For this review, use the dimensioned drawing (mm, ordinates from the lowest corner) and the shaded views. A direction names the side the tool comes from. Round coordinates to 2 decimals unless told otherwise and drop trailing zeros. Write each loop counter-clockwise with the first axis right and the second up, starting at its lowest first coordinate (ties: lowest second). Pieces come first, ordered by that corner, then holes. Notation, with made-up numbers: M 78.25,33.5 L 129.25,33.5 A11 cw 129.25,54.5 Z; hole C 25.5,14 d6. An arc over 180 degrees is marked long. Use CSV: the item, a comma, the result in double quotes.
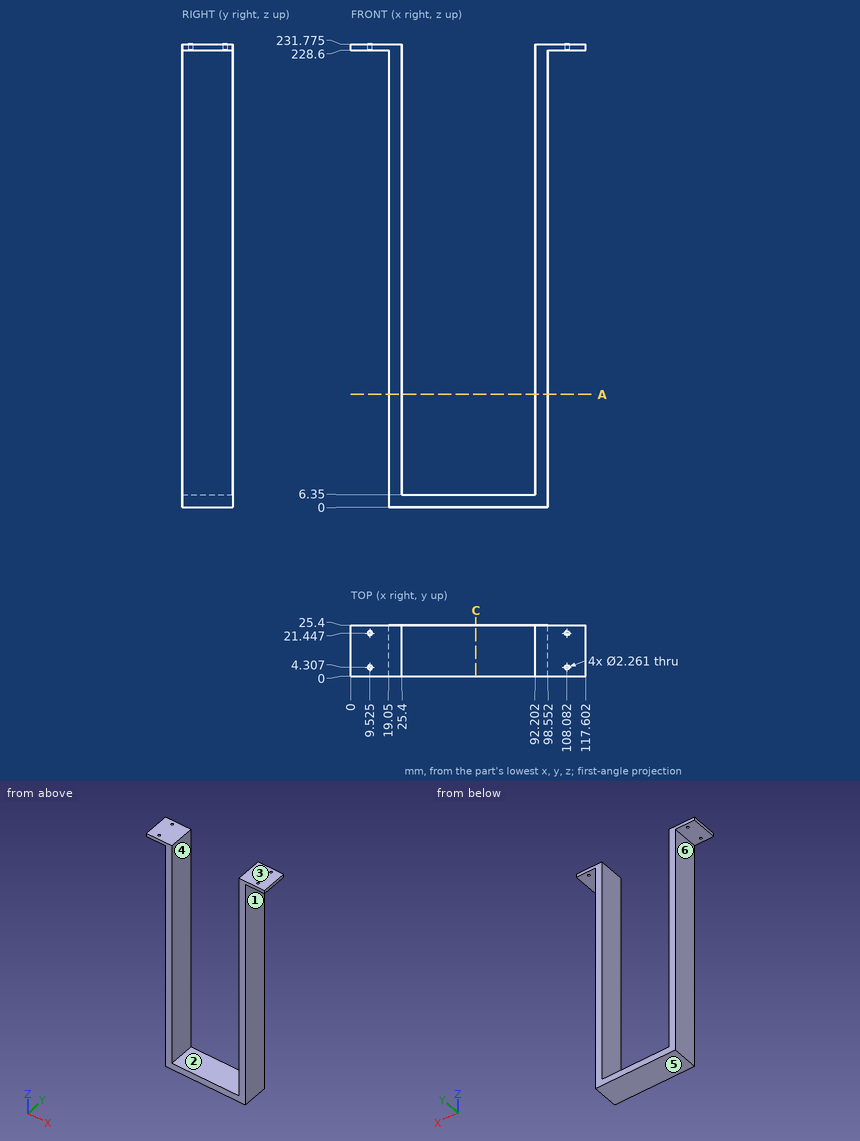
1) Wall thickness on line 1 along X through (y, z) = (22.75, 179.5); line 2 along Z through (x, y) = (62.5, 3.5); line 3 along Z through (x, y) = (99, 19.75) (1 decimal): over which ranges is each line inside the solid? List them lowest first. Write a range as [from, to].
Answers:
line 1,"[19.05, 25.4], [92.2, 98.55]"
line 2,"[0, 6.35]"
line 3,"[228.6, 231.8]"
2) Machinability: for the marked faces 1, 2 and 3, which of the approach directions +Z, -Z, +X, -X, +Y, -Y give a long, thin tool a straight path to every point of the face, cutting with its end or side? Answer none if there is none.
Answers:
face 1,"-Z, +X, +Y, -Y"
face 2,"+Z, +Y, -Y"
face 3,"+Z, +X, -X, +Y, -Y"
3) Add section A-A on z = 56.5. Write out the cut boundary in (x, y).
Answers:
outline,"M 19.05,0 L 25.4,0 L 25.4,25.4 L 19.05,25.4 Z; M 92.2,0 L 98.55,0 L 98.55,25.4 L 92.2,25.4 Z"
4) Add section C-C on x = 62.5. Write out the cut boundary in (y, z).
Answers:
outline,"M 0,0 L 25.4,0 L 25.4,6.35 L 0,6.35 Z"
5) For pin 1 Ø4 at (y, z) = (14, 124) entering from -X; pin 2 Ø3.5 at (x, y) = (108.08, 21.45) entering from -Z; pin 3 Ø7.5 at (y, z) = (15.5, 63) entering from +X, all flat-tipped, find the tip position at first contact; note any pin that passes through.
Answers:
pin 1,"x = 19.05"
pin 2,"z = 228.6"
pin 3,"x = 98.55"
6) The part is to be moulded in two halves that separate along X. For the marked faces 4, 5 and 6, say which applies: released by +X, released by -X, zero draft, split by the parting line, or undercut.
Answers:
face 4,"undercut"
face 5,"zero draft"
face 6,"released by -X"
